Geometry: final body of the model. Coordinates: model frame, mm. A direction names the side the tool comes from. Give positions to 0.01 mm unless a question says otherwise; leave off trailing zeros. Loops run counter-clockwise (first coordinate to the right, second up) from the corner with the lowest first, then second, coordinate; pieces in that order, holes last. Notation, with made-up numbers: (-19.75, 70.5) - (-5.75, 70.5) arc R19 cw to (-5.75, 74.5) - close; hole circle Ø6 at (-26.75, 24). An arc over 180 degrees is marked (long way). Use one line per item in the form item = value.
```python
from build123d import *

# Parameters (mm, degrees)
BOSS_EXTRUDE1_DEPTH     = 22.098
CUT_EXTRUDE1_DEPTH      = 11.2522
M10X1_5_TAPPED_HOLE1_D  = 8.5
SKETCH6_R               = 6.4135
CUT_EXTRUDE2_DEPTH      = 54.169790332
F_1_4_28_TAPPED_HOLE1_D = 5.4102


with BuildPart() as part:
    # Sketch1 → Boss-Extrude1 (new body)
    with BuildSketch(Plane(origin=(0, 0, 0), x_dir=(1, 0, 0), z_dir=(0, 1, 0))):
        Polygon((-44.45, -6.35), (-25.4, -19.05), (25.4, -19.05), (44.45, -6.35), (44.45, 19.05), (-44.45, 19.05), align=None)
    extrude(amount=BOSS_EXTRUDE1_DEPTH)

    # Sketch2 → Cut-Extrude1 (cut)
    with BuildSketch(Plane(origin=(0, 22.098, 0), x_dir=(1, 0, 0), z_dir=(0, 1, 0))):
        with BuildLine():
            Line((-31.75, 19.05), (-31.75, 9.525))
            ThreePointArc((-31.75, 9.525), (-32.67993597, 7.27993597), (-34.925, 6.35))
            Line((-34.925, 6.35), (-44.45, 6.35))
            Line((-44.45, 6.35), (-44.45, 19.05))
            Line((-44.45, 19.05), (-31.75, 19.05))
        make_face()
    extrude(amount=-CUT_EXTRUDE1_DEPTH, mode=Mode.SUBTRACT)

    # M10x1.5 Tapped Hole1 (through all)
    with Locations(Plane.XY.offset(19.05)):
        with Locations((0, 11.049)):
            Hole(M10X1_5_TAPPED_HOLE1_D / 2)

    # Sketch6 → Cut-Extrude2 (cut, through all)
    with BuildSketch(Plane(origin=(0, 22.098, 0), x_dir=(1, 0, 0), z_dir=(0, 1, 0))):
        with Locations(Location((-17.4625, 3.364454491, 0), (0, 0, 270))):
            Circle(SKETCH6_R)
        with Locations(Location((17.4625, 3.364454491, 0), (0, 0, 90))):
            Circle(SKETCH6_R)
    extrude(amount=-CUT_EXTRUDE2_DEPTH, mode=Mode.SUBTRACT)

    # 1/4-28 Tapped Hole1 (through all)
    with Locations(Plane.XZ):
        with Locations((-17.4625, 15.685545509)):
            Hole(F_1_4_28_TAPPED_HOLE1_D / 2)


solid = part.part
```
(1) Cut plane B-B (x = 0). Return the cut outline in (y, z).
Solution:
outline = (0, -19.05) - (6.8, -19.05) - (6.8, 19.05) - (0, 19.05) - close; (15.3, -19.05) - (22.1, -19.05) - (22.1, 19.05) - (15.3, 19.05) - close
(2) Access query for faces 1 (the face through (-1, 22.098, 0)), 2 (the face through (-33, 17, -7)). Directions: +Z, -Z, +X, -X, +Y, -Y. A direction counts if a zero-diameter tool reaches every point of the face in a straight line with its end or side. Return the directions, or none.
Solution:
face_1 = +Z, -Z, +X, -X, +Y
face_2 = -Z, -X, +Y
(3) Pin query (flat end, axial travel): P1, Ø7.5, axis at y = 18, z = -12, coming from the -X side; P2, Ø6.5, axis at x = -37.5, z = -14, coming from the +Y side; P3, Ø5, axis at x = -39, y = 15.5, coming from the -Z side. Return the tip coordinate at first contact, or that it passes through.
Solution:
P1 = -32.02
P2 = 10.85
P3 = -6.35
(4) Cut plane C-C (y = 8.75). Return the cut outline in (x, z), plus the area to 3 significant figures.
Solution:
outline = (-44.45, -19.05) - (-3.57, -19.05) - (-3.57, 19.05) - (-25.4, 19.05) - (-44.45, 6.35) - close; (3.57, -19.05) - (44.45, -19.05) - (44.45, 6.35) - (25.4, 19.05) - (3.57, 19.05) - close; hole circle Ø12.83 at (-17.46, -3.36); hole circle Ø5.41 at (-17.46, 15.69); hole circle Ø12.83 at (17.46, -3.36)
area = 2,590 mm2
(5) Material intervals for L1, parallel to Y at x = 0, z = -8.5; L2, parallel to Z at x = -15.5, y = 16.75; L3, parallel to X at y = 14, z = 7 (3 decimals), sorted ascending. Write a range as from..to.
Solution:
L1 = 0..6.8, 15.3..22.1
L2 = -19.05..-9.47, 2.74..13.82, 17.55..19.05
L3 = -43.475..-3.058, 3.058..43.475
(6) Cut plane D-D (z = 1.5). Return the cut outline in (x, y), plus the area to 3 significant figures.
Solution:
outline = (-44.45, 0) - (-21.64, 0) - (-21.64, 22.1) - (-44.45, 22.1) - close; (-13.28, 0) - (13.28, 0) - (13.28, 22.1) - (-13.28, 22.1) - close; (21.64, 0) - (44.45, 0) - (44.45, 22.1) - (21.64, 22.1) - close; hole circle Ø8.5 at (0, 11.05)
area = 1,540 mm2
(7) Pull-direction query (X, two-part tool) for faces 3 (the face through (-15.316, 11.204, 14.04)), 4 (the face through (-15.536, 11.204, 2.753)), 5 (the face through (-1, 0, 0)), 6 (the face through (-35.06, 10.89, 12.61)); classes: released by +X, released by -X, zero draft, split by the parting line, or undercut.
Solution:
face_3 = undercut
face_4 = undercut
face_5 = zero draft
face_6 = released by -X
(8) Cut plane A-A (z = -14). Return the cut outline in (x, y).
Solution:
outline = (-44.45, 0) - (44.45, 0) - (44.45, 22.1) - (-31.75, 22.1) - (-31.75, 10.85) - (-44.45, 10.85) - close; hole circle Ø8.5 at (0, 11.05)
